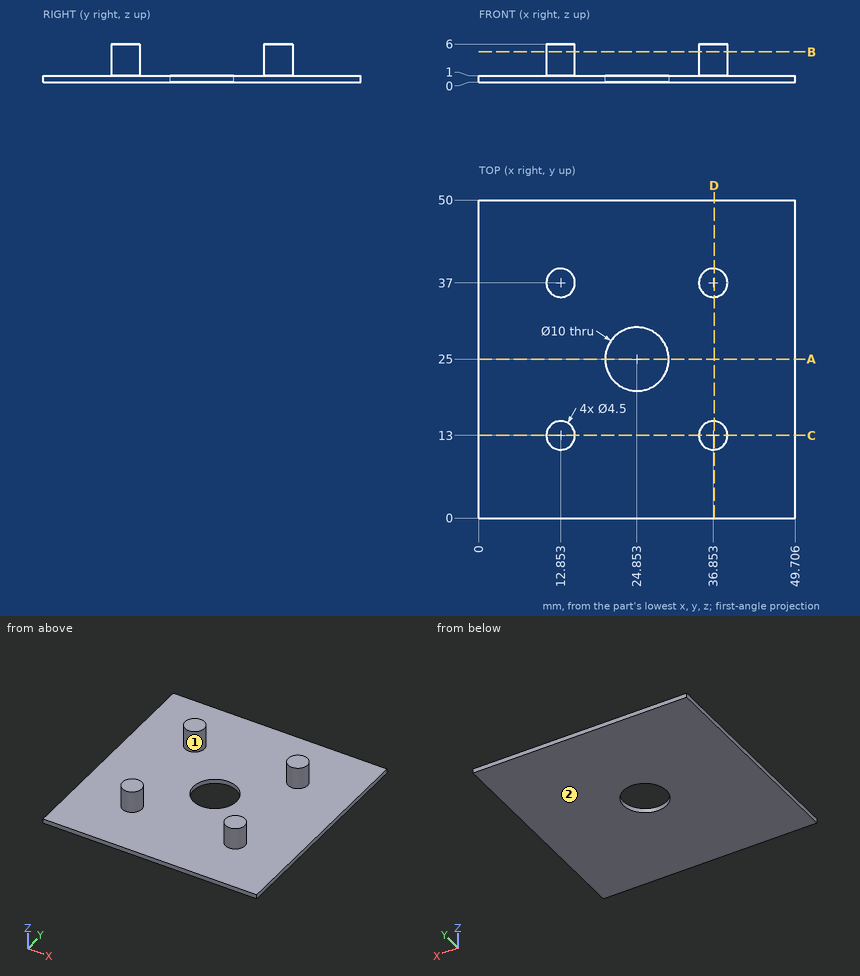
Design review of the part shown in the three views and the two pictorial views. Dimensions are in mm from the part's minimum x, y and z. Round coordinates to 2 decimals unless told otherwise and drop trailing zeros. Order: outer loops, then holes, each group sorted by start corner. A loop starts at its lowest first (then second) coordinate and runs counter-clockwise, first axis right, second up.
(1) Take a section at A-A, the plane y = 25. State the section outline as (x, z) points, plus the area to 3 significant figures.
Working result:
outline: (0, 0) - (19.85, 0) - (19.85, 1) - (0, 1) - close; (29.85, 0) - (49.71, 0) - (49.71, 1) - (29.85, 1) - close
area: 39.7 mm2
(2) Take a section at B-B, the plane z = 4.75. State the section outline as (x, y) points.
Working result:
outline: circle Ø4.5 at (12.85, 13); circle Ø4.5 at (12.85, 37); circle Ø4.5 at (36.85, 13); circle Ø4.5 at (36.85, 37)
(3) Take a section at C-C, the plane y = 13. State the section outline as (x, z) points, plus the area to 3 significant figures.
Working result:
outline: (0, 0) - (49.71, 0) - (49.71, 1) - (39.1, 1) - (39.1, 6) - (34.6, 6) - (34.6, 1) - (15.1, 1) - (15.1, 6) - (10.6, 6) - (10.6, 1) - (0, 1) - close
area: 94.7 mm2
(4) For P1, Ø5, axis at x = 28.5, y = 11, coming from the +Z side; P2, Ø3, axis at x = 28, y = 23, coming from the -Z side, all flat-tipped, find the tip position at first contact; note any pin that passes through.
Working result:
P1: stops at z = 1
P2: stops at z = 0
(5) Take a section at D-D, the plane x = 37. State the section outline as (y, z) points, plus the area to 3 significant figures.
Working result:
outline: (0, 0) - (50, 0) - (50, 1) - (39.25, 1) - (39.25, 6) - (34.75, 6) - (34.75, 1) - (15.25, 1) - (15.25, 6) - (10.75, 6) - (10.75, 1) - (0, 1) - close
area: 94.9 mm2
(6) Mouldability with a two-part tool opening along Y and no side actions: class the marked faces 1 and 2 as released by +Y, released by -Y, zero draft, split by the parting line, or undercut.
Working result:
face 1: undercut
face 2: zero draft
(7) Wall thickness on L1, parallel to Z at x = 5.5, y = 11.5; L2, parallel to X at y = 14, z = 2.35; L3, parallel to Y at x = 36.5, z = 1.35: over which ranges is each line inside the solid? List them lowest first.
Working result:
L1: z = 0 to 1
L2: x = 10.84 to 14.87, 34.84 to 38.87
L3: y = 10.78 to 15.22, 34.78 to 39.22
